```python
from build123d import *

# Parameters (mm, degrees)
ESBO_O1_W                = 80
ESBO_O1_H                = 130
RESSALTO_EXTRUS_O1_DEPTH = 15
ESBO_O2_R                = 7.7
CORTE_EXTRUS_O1_DEPTH    = 16
ESBO_O3_R                = 9.7
CORTE_EXTRUS_O2_DEPTH    = 12
ESBO_O4_R                = 4.6
CORTE_EXTRUS_O3_DEPTH    = 4
ESBO_O5_W                = 15
ESBO_O5_H                = 20
ESBO_O5_W_2              = 20
ESBO_O5_H_2              = 15
CORTE_EXTRUS_O4_DEPTH    = 16
ESBO_O6_R                = 2.4
CORTE_EXTRUS_O5_DEPTH    = 15
ESBO_O7_R                = 2.4
CORTE_EXTRUS_O6_DEPTH    = 15
ESBO_O8_R                = 11
CORTE_EXTRUS_O7_DEPTH    = 3
ESBO_O10_R               = 5.1
ESBO_O10_R_2             = 1.5
CORTE_EXTRUS_O9_DEPTH    = 13
FILETE1_R                = 5
FILETE2_R                = 5
ESBO_O11_R               = 2.4
CORTE_EXTRUS_O10_DEPTH   = 15
CORTE_EXTRUS_O11_DEPTH   = 4
CORTE_EXTRUS_O12_DEPTH   = 4
CORTE_EXTRUS_O13_DEPTH   = 4


with BuildPart() as part:
    # Esboço1 → Ressalto-extrusão1 (new body)
    with BuildSketch(Plane(origin=(0, 0, 0), x_dir=(1, 0, 0), z_dir=(0, 1, 0))):
        Rectangle(ESBO_O1_W, ESBO_O1_H)
    extrude(amount=RESSALTO_EXTRUS_O1_DEPTH)

    # Esboço2 → Corte-extrusão1 (cut, through all)
    with BuildSketch(Plane(origin=(0, 15, 0), x_dir=(1, 0, 0), z_dir=(0, 1, 0))):
        with Locations((-30, 5)):
            Circle(ESBO_O2_R)
        with Locations((30, 5)):
            Circle(ESBO_O2_R)
        with Locations((-30, -55)):
            Circle(ESBO_O2_R)
        with Locations((30, -55)):
            Circle(ESBO_O2_R)
        with Locations((-30, 40)):
            Circle(ESBO_O2_R)
        with Locations((30, 40)):
            Circle(ESBO_O2_R)
    extrude(amount=-CORTE_EXTRUS_O1_DEPTH, mode=Mode.SUBTRACT)

    # Esboço3 → Corte-extrusão2 (cut)
    with BuildSketch(Plane(origin=(0, 15, 0), x_dir=(1, 0, 0), z_dir=(0, 1, 0))):
        with Locations((0, -25)):
            Circle(ESBO_O3_R)
    extrude(amount=-CORTE_EXTRUS_O2_DEPTH, mode=Mode.SUBTRACT)

    # Esboço4 → Corte-extrusão3 (cut, through all)
    with BuildSketch(Plane(origin=(0, 3, 0), x_dir=(1, 0, 0), z_dir=(0, 1, 0))):
        with Locations((0, -25)):
            Circle(ESBO_O4_R)
    extrude(amount=-CORTE_EXTRUS_O3_DEPTH, mode=Mode.SUBTRACT)

    # Esboço5 → Corte-extrusão4 (cut, through all)
    with BuildSketch(Plane(origin=(0, 15, 0), x_dir=(1, 0, 0), z_dir=(0, 1, 0))):
        with Locations((0, -55)):
            Rectangle(ESBO_O5_W, ESBO_O5_H)
        with Locations((30, -25)):
            Rectangle(ESBO_O5_W_2, ESBO_O5_H_2)
        with Locations((-30, -25)):
            Rectangle(ESBO_O5_W_2, ESBO_O5_H_2)
    extrude(amount=-CORTE_EXTRUS_O4_DEPTH, mode=Mode.SUBTRACT)

    # Esboço6 → Corte-extrusão5 (cut)
    with BuildSketch(Plane.XY.offset(45)):
        with Locations((0, 9)):
            Circle(ESBO_O6_R)
    extrude(amount=-CORTE_EXTRUS_O5_DEPTH, mode=Mode.SUBTRACT)

    # Esboço7 → Corte-extrusão6 (cut)
    with BuildSketch(Plane(origin=(20, 0, 0), x_dir=(0, 0, -1), z_dir=(1, 0, 0))):
        with Locations((-25, 9)):
            Circle(ESBO_O7_R)
    extrude(amount=-CORTE_EXTRUS_O6_DEPTH, mode=Mode.SUBTRACT)

    # Esboço8 → Corte-extrusão7 (cut)
    with BuildSketch(Plane(origin=(0, 15, 0), x_dir=(1, 0, 0), z_dir=(0, 1, 0))):
        with Locations((0, 40)):
            Circle(ESBO_O8_R)
    extrude(amount=-CORTE_EXTRUS_O7_DEPTH, mode=Mode.SUBTRACT)

    # Esboço10 → Corte-extrusão9 (cut, through all)
    with BuildSketch(Plane(origin=(0, 12, 0), x_dir=(1, 0, 0), z_dir=(0, 1, 0))):
        with Locations((0, 40)):
            Circle(ESBO_O10_R)
        with Locations((0, 48)):
            Circle(ESBO_O10_R_2)
        with Locations((8, 40)):
            Circle(ESBO_O10_R_2)
        with Locations((0, 32)):
            Circle(ESBO_O10_R_2)
        with Locations((-8, 40)):
            Circle(ESBO_O10_R_2)
    extrude(amount=-CORTE_EXTRUS_O9_DEPTH, mode=Mode.SUBTRACT)

    # Filete1
    filete1_edges = [part.edges().sort_by_distance(p)[0] for p in [
        (-40, 7.5, -65),
        (40, 7.5, -65),
    ]]
    fillet(filete1_edges, radius=FILETE1_R)

    # Filete2
    filete2_edges = [part.edges().sort_by_distance(p)[0] for p in [
        (40, 7.5, 65),
        (-40, 7.5, 65),
    ]]
    fillet(filete2_edges, radius=FILETE2_R)

    # Esboço11 → Corte-extrusão10 (cut)
    with BuildSketch(Plane.ZY.offset(20)):
        with Locations((25, 9)):
            Circle(ESBO_O11_R)
    extrude(amount=-CORTE_EXTRUS_O10_DEPTH, mode=Mode.SUBTRACT)

    # Esboço12 → Corte-extrusão11 (cut)
    with BuildSketch(Plane.ZY.offset(17)):
        Polygon((22.75, 5.102885683), (27.25, 5.102885683), (29.5, 9), (29.5, 15), (20.5, 15), (20.5, 9), align=None)
    extrude(amount=-CORTE_EXTRUS_O11_DEPTH, mode=Mode.SUBTRACT)

    # Esboço13 → Corte-extrusão12 (cut)
    with BuildSketch(Plane.XY.offset(42)):
        Polygon((-2.25, 5.102885683), (2.25, 5.102885683), (4.5, 9), (4.5, 15), (-4.5, 15), (-4.5, 9), align=None)
    extrude(amount=-CORTE_EXTRUS_O12_DEPTH, mode=Mode.SUBTRACT)

    # Esboço14 → Corte-extrusão13 (cut)
    with BuildSketch(Plane(origin=(17, 0, 0), x_dir=(0, 0, -1), z_dir=(1, 0, 0))):
        Polygon((-27.25, 5.102885683), (-22.75, 5.102885683), (-20.5, 9), (-20.5, 15), (-29.5, 15), (-29.5, 9), align=None)
    extrude(amount=-CORTE_EXTRUS_O13_DEPTH, mode=Mode.SUBTRACT)


solid = part.part
```
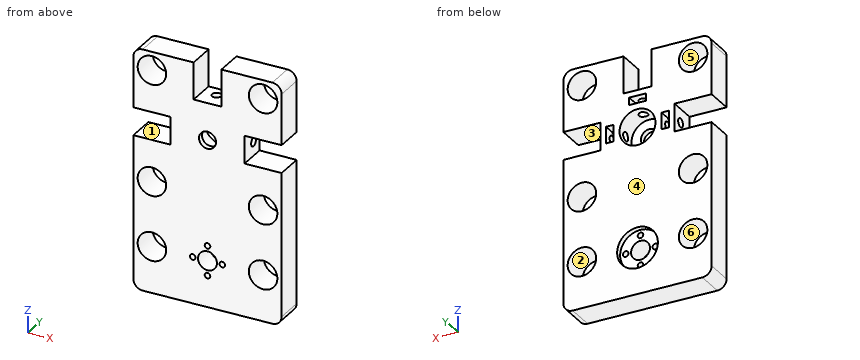
For this review, take the finished solid that the model builds, in its own axes (mm). Face numbers are marked on the shaded views. A direction names the side the tool comes from. Coordinates: 2 decimals unless noted, no trailing zeros. Write each loop counter-clockwise with the first axis right and the second up, starting at its lowest first coordinate (ties: lowest second). Pieces come first, ordered by that corner, then holes. Notation, with made-up numbers: (37, -10) - (86, -10) arc R23 ccw to (86, 27) - close; hole circle Ø3 at (87.5, 1.25). An arc over 180 degrees is marked (long way). Answer in a Markdown table with one row per item. Add a question column.
Q1. For P1, Ø1.2, axis at x = -15, z = 26, coming from the +Y side; P2, Ø2.5, axis at x = 0, z = -48, coming from the -Y side; P3, Ø7.5, axis at y = 7, z = 23, coming from the +X side, all flat-tipped, find the tip position at first contact; note any pin that passes through.
Q2. For probe 1 along X at (y, z) = (10.25, -40); probe 2 along Z at (x, y) = (30, 11.75); probe 3 along X at (y, z) = (8.75, -5), list the stretches that pass through material, from the lowest coordinate up.
Q3. Tool access review of the marked faces 1, 2 and 3: name each direction out of +Z, -Z, +X, -X, +Y, -Y from which nothing blocks a thin tool from reaching the whole face with its end or side.
Q4. We need section A-A, the plane z = -40. State the section outline as (x, y) points, and give its area (3 significant figures).
Q5. Draft analysis for pull direction X (two halves, no side actions). For the marked faces 4, 5 and 6, state which applies: +X half, -X half, draft (parallel to the pull), parting line (faces both ways), or undercut.
Q6. We need section C-C, the plane x = -30. State the section outline as (y, z) points, and give its area (3 significant figures).
Q7. We need section B-B, the plane y = 1.5. Count the separate pieces of the cut face and the enclosed holes in it, and give its area (3 significant figures).
Answer list:
| question | item | result |
|---|---|---|
| 1 | P1 | stops at y = 5.1 |
| 1 | P2 | passes through |
| 1 | P3 | stops at x = 20 |
| 2 | probe 1 | x = -40 to -37.7, -22.3 to -9.5, -6.5 to -5.1, 5.1 to 6.5, 9.5 to 22.3, 37.7 to 40 |
| 2 | probe 2 | z = -65 to -47.7, -32.3 to -12.7, 2.7 to 17.5, 32.5 to 47.3, 62.7 to 65 |
| 2 | probe 3 | x = -40 to -37.7, -22.3 to 22.3, 37.7 to 40 |
| 3 | face 1 | -X, +Y, -Y |
| 3 | face 2 | +Y, -Y |
| 3 | face 3 | +X, +Y, -Y |
| 4 | outline | (-40, 0) - (-37.7, 0) - (-37.7, 15) - (-40, 15) - close; (-22.3, 0) - (-9.5, 0) - (-9.5, 12) - (-11, 12) - (-11, 15) - (-22.3, 15) - close; (-6.5, 0) - (-5.1, 0) - (-5.1, 12) - (-6.5, 12) - close; (5.1, 0) - (6.5, 0) - (6.5, 12) - (5.1, 12) - close; (9.5, 0) - (22.3, 0) - (22.3, 15) - (11, 15) - (11, 12) - (9.5, 12) - close; (37.7, 0) - (40, 0) - (40, 15) - (37.7, 15) - close |
| 4 | area | 478 mm2 |
| 5 | face 4 | draft |
| 5 | face 5 | undercut |
| 5 | face 6 | undercut |
| 6 | outline | (0, -65) - (15, -65) - (15, -47.7) - (0, -47.7) - close; (0, -32.3) - (15, -32.3) - (15, -12.7) - (0, -12.7) - close; (0, 2.7) - (15, 2.7) - (15, 17.5) - (0, 17.5) - close; (0, 32.5) - (15, 32.5) - (15, 47.3) - (0, 47.3) - close; (0, 62.7) - (15, 62.7) - (15, 65) - (0, 65) - close |
| 6 | area | 1,030 mm2 |
| 7 | separate pieces | 1 |
| 7 | enclosed holes | 12 |
| 7 | area | 8,180 mm2 |
